```python
from build123d import *

# Parameters (mm, degrees)
SKETCH2_W             = 53
SKETCH2_H             = 49
BOSS_EXTRUDE1_DEPTH   = 36.4
SKETCH3_W             = 11.5
SKETCH3_H             = 18.2
CUT_EXTRUDE1_DEPTH    = 50
CHAMFER1_SIZE         = 10
CHAMFER1_SIZE2        = 7.002075382
CHAMFER2_SIZE         = 2
CHAMFER2_SIZE2        = 1.400415076
CHAMFER2_PART_2_SIZE  = 2
CHAMFER2_PART_2_SIZE2 = 1.400415076
CHAMFER2_PART_3_SIZE  = 2
CHAMFER2_PART_3_SIZE2 = 1.400415076
CHAMFER2_PART_4_SIZE  = 2
CHAMFER2_PART_4_SIZE2 = 1.400415076
SKETCH4_R             = 3.5
BOSS_EXTRUDE2_DEPTH   = 10
SKETCH5_R             = 4
CUT_EXTRUDE2_DEPTH    = 10


with BuildPart() as part:
    # Sketch2 → Boss-Extrude1 (new body)
    with BuildSketch(Plane(origin=(0, 0, 0), x_dir=(1, 0, 0), z_dir=(0, 1, 0))):
        Rectangle(SKETCH2_W, SKETCH2_H)
    extrude(amount=BOSS_EXTRUDE1_DEPTH)

    # Sketch3 → Cut-Extrude1 (cut, through all)
    with BuildSketch(Plane.XY.offset(24.5)):
        with Locations((-20.75, 27.3)):
            Rectangle(SKETCH3_W, SKETCH3_H)
        with Locations((20.75, 27.3)):
            Rectangle(SKETCH3_W, SKETCH3_H)
    extrude(amount=-CUT_EXTRUDE1_DEPTH, mode=Mode.SUBTRACT)

    # Chamfer1
    chamfer1_edges = [part.edges().sort_by_distance(p)[0] for p in [
        (0, 36.4, 24.5),
        (0, 36.4, -24.5),
    ]]
    chamfer1_side = [part.faces().sort_by_distance(p)[0] for p in [
        (0, 36.4, 0),
    ]]
    chamfer(chamfer1_edges, length=CHAMFER1_SIZE, length2=CHAMFER1_SIZE2, reference=chamfer1_side[0])

    # Chamfer2
    chamfer2_edges = [part.edges().sort_by_distance(p)[0] for p in [
        (-26.5, 9.1, -24.5),
    ]]
    chamfer2_side = [part.faces().sort_by_distance(p)[0] for p in [
        (0, 12.896841884, -24.5),
    ]]
    chamfer(chamfer2_edges, length=CHAMFER2_SIZE, length2=CHAMFER2_SIZE2, reference=chamfer2_side[0])

    # Chamfer2 part 2
    chamfer2_part_2_edges = [part.edges().sort_by_distance(p)[0] for p in [
        (26.5, 9.1, -24.5),
    ]]
    chamfer2_part_2_side = [part.faces().sort_by_distance(p)[0] for p in [
        (26.5, 9.1, 0),
    ]]
    chamfer(chamfer2_part_2_edges, length=CHAMFER2_PART_2_SIZE, length2=CHAMFER2_PART_2_SIZE2, reference=chamfer2_part_2_side[0])

    # Chamfer2 part 3
    chamfer2_part_3_edges = [part.edges().sort_by_distance(p)[0] for p in [
        (26.5, 9.1, 24.5),
    ]]
    chamfer2_part_3_side = [part.faces().sort_by_distance(p)[0] for p in [
        (0, 12.896841884, 24.5),
    ]]
    chamfer(chamfer2_part_3_edges, length=CHAMFER2_PART_3_SIZE, length2=CHAMFER2_PART_3_SIZE2, reference=chamfer2_part_3_side[0])

    # Chamfer2 part 4
    chamfer2_part_4_edges = [part.edges().sort_by_distance(p)[0] for p in [
        (-26.5, 9.1, 24.5),
    ]]
    chamfer2_part_4_side = [part.faces().sort_by_distance(p)[0] for p in [
        (-26.5, 9.1, 0),
    ]]
    chamfer(chamfer2_part_4_edges, length=CHAMFER2_PART_4_SIZE, length2=CHAMFER2_PART_4_SIZE2, reference=chamfer2_part_4_side[0])

    # Sketch4 → Boss-Extrude2 (add)
    with BuildSketch(Plane(origin=(0, 18.2, 0), x_dir=(1, 0, 0), z_dir=(0, 1, 0))):
        with Locations((20.75, -18.75)):
            Circle(SKETCH4_R)
        with Locations((20.75, 18.75)):
            Circle(SKETCH4_R)
    extrude(amount=BOSS_EXTRUDE2_DEPTH)

    # Sketch5 → Cut-Extrude2 (cut)
    with BuildSketch(Plane(origin=(0, 18.2, 0), x_dir=(1, 0, 0), z_dir=(0, 1, 0))):
        with Locations((-20.75, 15.299792462)):
            Circle(SKETCH5_R)
        with Locations((-20.75, -14.700207538)):
            Circle(SKETCH5_R)
        with Locations((-20.75, 0.299792462)):
            Circle(SKETCH5_R)
    extrude(amount=-CUT_EXTRUDE2_DEPTH, mode=Mode.SUBTRACT)


solid = part.part
```
Model file for the job. Use its own axes, mm. A direction names the side the tool comes from. Give positions to 0.01 mm unless a question says otherwise; leave off trailing zeros. Write each loop counter-clockwise with the first axis right and the second up, starting at its lowest first coordinate (ties: lowest second). Pieces come first, ordered by that corner, then holes. Notation, with made-up numbers: M 73.5,-13.75 L 121.5,-13.75 A21 ccw 121.5,-1.75 Z; hole C 28.25,58 d1. An arc over 180 degrees is marked long. Use a Markdown table: item, result.
1) Pull direction X, two halves, no side cores. Call faces 1 (the flat face through (-0.21, 32.85, 19.57)), 2 (the cylindrical face through (22.63, 23.13, 15.8)), 3 (the flat face through (-15, 27, 0)): +X half, -X half, draft (parallel to the pull), parting line (faces both ways), or undercut.
Responses:
| item | result |
|---|---|
| face 1 | draft |
| face 2 | undercut |
| face 3 | -X half |
2) Cut at D-D (y = 15.5). List the corners of the cut face in (x, z).
Responses:
| item | result |
|---|---|
| outline | M -26.5,-23.1 L -24.5,-24.5 L 25.1,-24.5 L 26.5,-22.5 L 26.5,23.1 L 24.5,24.5 L -25.1,24.5 L -26.5,22.5 Z; hole C -20.75,-15.3 d8; hole C -20.75,-0.3 d8; hole C -20.75,14.7 d8 |
3) Cut at A-A (y = 20). List the corners of the cut face in (x, z).
Responses:
| item | result |
|---|---|
| outline | M -15,-24.5 L 15,-24.5 L 15,24.5 L -15,24.5 Z; C 20.75,-18.75 d7; C 20.75,18.75 d7 |
4) Cut at C-C (z = -9.5). List the corners of the cut face in (x, y).
Responses:
| item | result |
|---|---|
| outline | M -26.5,0 L 26.5,0 L 26.5,18.2 L 15,18.2 L 15,36.4 L -15,36.4 L -15,18.2 L -26.5,18.2 Z |
5) Tool access for faces 4 (the flat face through (-25.5, 9, -23.8)), 5 (the flat face through (15, 27, 0)), 6 (the flat face through (21, 18.2, 0)), 7 (the flat face through (21, 28.2, 19)): list every direction of +Z, -Z, +X, -X, +Y, -Y with a clear straight run to the whole face (end or side of a thin tool).
Responses:
| item | result |
|---|---|
| face 4 | -Z, -X, +Y, -Y |
| face 5 | +Z, -Z, +Y |
| face 6 | +Y |
| face 7 | +Z, -Z, +X, +Y |
6) Cut at B-B (x = -20.75). List the corners of the cut face in (y, z), and give its area (3 significant figures).
Responses:
| item | result |
|---|---|
| outline | M 0,-24.5 L 18.2,-24.5 L 18.2,-19.3 L 8.2,-19.3 L 8.2,-11.3 L 18.2,-11.3 L 18.2,-4.3 L 8.2,-4.3 L 8.2,3.7 L 18.2,3.7 L 18.2,10.7 L 8.2,10.7 L 8.2,18.7 L 18.2,18.7 L 18.2,24.5 L 0,24.5 Z |
| area | 652 mm2 |
7) Pin check, flat tips, straight feed: pin 1 (7 mm diameter, centred on x = -20.75, z = 14.7, fed in from -Y); pin 2 (6.5 mm diameter, centred on x = -19.5, z = -16, fed in from +Y); pin 3 (5.5 mm diameter, centred on x = 21.5, z = 17.5, fed in from +Y); pin 4 (1 mm diameter, centred on x = 8.5, y = 30.5, fed in from -Z). Stop position of each tip, or through.
Responses:
| item | result |
|---|---|
| pin 1 | stops at y = 0 |
| pin 2 | stops at y = 18.2 |
| pin 3 | stops at y = 28.2 |
| pin 4 | stops at z = -23.64 |
8) Drill centre lines: line 1 (Z direction, x = -20.75, y = 15.5); line 2 (Y direction, x = 21, z = 22.5); line 3 (X direction, y = 31, z = -19). Where is each one in solid material? Low to high. Write a range as from..to.
Responses:
| item | result |
|---|---|
| line 1 | z = -24.5..-19.3, -11.3..-4.3, 3.7..10.7, 18.7..24.5 |
| line 2 | y = 0..18.2 |
| line 3 | x = -15..15 |
